```python
from build123d import *

# Parameters (mm, degrees)
F1_DEPTH = 4.5
F1_TAPER = 3
F2_R     = 2.5
F3_DEPTH = 25
F4_SIZE  = 0.3


with BuildPart() as f1:
    # F0 (on Top) → F1 (new body)
    with BuildSketch(Plane.XY):
        Polygon((-1.2996787849, -4), (1.2996787849, -4), (3.4026032334, -2.472135955), (4.205848897, 0), (3.4026032334, 2.472135955), (1.2996787849, 4), (-1.2996787849, 4), (-3.4026032334, 2.472135955), (-4.205848897, 0), (-3.4026032334, -2.472135955), align=None)
    extrude(amount=F1_DEPTH, taper=F1_TAPER)

    # F2 (on face) → F3 (cut)
    with BuildSketch(Plane.XY.offset(4.5)):
        Circle(F2_R)
    extrude(amount=-F3_DEPTH, mode=Mode.SUBTRACT)

    # F4
    f4_edges = [f1.edges().sort_by_distance(p)[0] for p in [
        (-2.5, 0, 4.5),
        (-2.5, 0, 0),
    ]]
    chamfer(f4_edges, length=F4_SIZE)


solid = f1.part
```
Can you work these out from the model? Positions are in its coordinate system, mm. Round coordinates to 2 decimals unless told otherwise and drop trailing zeros. Loops run counter-clockwise (first coordinate to the right, second up) from the corner with the lowest first, then second, coordinate; pieces in that order, holes last.
Item 1: Please list where these lines run through material, in increasing order: L1, parallel to X at y = -1, z = 2.7; L2, parallel to X at y = -0.75, z = 3.85; L3, parallel to Y at x = 0, z = 2.
Item 2: If we mould it in two halves opening along X, with no side actions, what happens to faces 1 (the flat face through (-0.018, 3.884, 2.219)), 2 (the cylindrical face through (-0.54, -2.44, 2.28)), 3 (the flat face through (-2.3, 3.13, 2.22)), 4 (the flat face through (2.3, -3.13, 2.22))? For each: +X half, -X half, draft (parallel to the pull), parting line (faces both ways), or undercut.
Item 3: Suppose I cut it at C-C, the plane z = 1.1. Write out the boundary of the cut face in (x, y).
Item 4: Suppose I cut it at B-B, the plane z = 3.55. Write out the boundary of the cut face in (x, y), then the cut area to 3 significant figures.
Item 5: Suppose I cut it at A-A, the plane x = 0. Write out the boundary of the cut face in (y, z).
Item 6: Will these pins go through, and if not, where does the flat tip stop? pin 1 Ø3 at (x, y) = (0, 0) entering from -Z; pin 2 Ø1.5 at (x, y) = (1.5, -1.5) entering from -Z; pin 3 Ø1.5 at (y, z) = (1, 4) entering from +X.
Reported:
1. L1: x = -3.73 to -2.29, 2.29 to 3.73
1. L2: x = -3.75 to -2.38, 2.38 to 3.75
1. L3: y = -3.9 to -2.5, 2.5 to 3.9
2. face 1: draft
2. face 2: undercut
2. face 3: -X half
2. face 4: +X half
3. outline: (-4.15, 0) - (-3.35, -2.44) - (-1.28, -3.94) - (1.28, -3.94) - (3.35, -2.44) - (4.15, 0) - (3.35, 2.44) - (1.28, 3.94) - (-1.28, 3.94) - (-3.35, 2.44) - close; hole circle Ø5 at (0, 0)
4. outline: (-4.01, 0) - (-3.24, -2.36) - (-1.24, -3.81) - (1.24, -3.81) - (3.24, -2.36) - (4.01, 0) - (3.24, 2.36) - (1.24, 3.81) - (-1.24, 3.81) - (-3.24, 2.36) - close; hole circle Ø5 at (0, 0)
4. area: 27.6 mm2
5. outline: (-4, 0) - (-2.8, 0) - (-2.5, 0.3) - (-2.5, 4.2) - (-2.8, 4.5) - (-3.76, 4.5) - close; (2.5, 0.3) - (2.8, 0) - (4, 0) - (3.76, 4.5) - (2.8, 4.5) - (2.5, 4.2) - close
6. pin 1: passes through
6. pin 2: stops at z = 0
6. pin 3: stops at x = 3.91
